from build123d import *

# Parameters (mm, degrees)
SKETCH2_W           = 350.52
SKETCH2_H           = 101.6
SKETCH2_R           = 43.18
SKETCH2_R_2         = 17.78
BOSS_EXTRUDE1_DEPTH = 15.24
SKETCH2_3_R         = 43.18
SKETCH2_3_R_2       = 20.32
BOSS_EXTRUDE2_DEPTH = 10.16
BOSS_EXTRUDE3_START = -50.8
BOSS_EXTRUDE3_DEPTH = 12.7
BOSS_EXTRUDE4_START = 50.8
BOSS_EXTRUDE4_DEPTH = 12.7
FILLET1_R           = 30.48


with BuildPart() as part:
    # Sketch2 → Boss-Extrude1 (new body)
    with BuildSketch(Plane(origin=(0, 0, 0), x_dir=(1, 0, 0), z_dir=(0, 1, 0))):
        Rectangle(SKETCH2_W, SKETCH2_H)
        Circle(SKETCH2_R, mode=Mode.SUBTRACT)
        with Locations((128.27, 0)):
            Circle(SKETCH2_R_2, mode=Mode.SUBTRACT)
        with Locations((-128.27, 0)):
            Circle(SKETCH2_R_2, mode=Mode.SUBTRACT)
    extrude(amount=BOSS_EXTRUDE1_DEPTH)

    # Sketch2<3> → Boss-Extrude2 (add)
    with BuildSketch(Plane(origin=(0, 0, 0), x_dir=(1, 0, 0), z_dir=(0, 1, 0))):
        Circle(SKETCH2_3_R)
        Circle(SKETCH2_3_R_2, mode=Mode.SUBTRACT)
    extrude(amount=BOSS_EXTRUDE2_DEPTH)

    # Sketch3 → Revolve1 (revolve)
    with BuildSketch(Plane.XY):
        Polygon((43.18, 15.24), (43.18, 0), (81.28, 0), (81.28, 101.6), (73.66, 101.6), (73.66, 96.52), (55.88, 96.52), (55.88, 71.12), (68.58, 71.12), (68.58, 15.24), align=None)
    revolve(axis=Axis((0, 0, 0), (0, 1, 0)))

    # Sketch4 → Boss-Extrude3 (add)
    with BuildSketch(Plane.XY.offset(BOSS_EXTRUDE3_START)):
        Polygon((119.38, 15.24), (63.297160251, 101.6), (63.297160251, 15.24), align=None)
        Polygon((-63.297160251, 15.24), (-119.38, 15.24), (-63.297160251, 101.6), align=None)
    extrude(amount=BOSS_EXTRUDE3_DEPTH)

    # Sketch4<2> → Boss-Extrude4 (add)
    with BuildSketch(Plane.XY.offset(BOSS_EXTRUDE4_START)):
        Polygon((119.38, 15.24), (63.297160251, 101.6), (63.297160251, 15.24), align=None)
        Polygon((-63.297160251, 15.24), (-119.38, 15.24), (-63.297160251, 101.6), align=None)
    extrude(amount=-BOSS_EXTRUDE4_DEPTH)

    # Fillet1
    fillet1_edges = [part.edges().sort_by_distance(p)[0] for p in [
        (-175.26, 7.62, 50.8),
        (-175.26, 7.62, -50.8),
        (175.26, 7.62, -50.8),
        (175.26, 7.62, 50.8),
    ]]
    fillet(fillet1_edges, radius=FILLET1_R)


solid = part.part
Model file for the job. Use its own axes, mm. A direction names the side the tool comes from. Give positions to 0.01 mm unless a question says otherwise; leave off trailing zeros. Loops run counter-clockwise (first coordinate to the right, second up) from the corner with the lowest first, then second, coordinate; pieces in that order, holes last.
Item 1: Drop flat-ended pins along their axis: P1, Ø3, axis at x = -58, y = 54, coming from the +Z side; P2, Ø5, axis at y = 73, z = -37.5, coming from the +X side; P3, Ø24.5, axis at x = -106, y = 27, coming from the +Z side. Give the stop position or say it passes through.
Check values:
P1: stops at z = 58.43
P2: stops at x = 83.45
P3: stops at z = 50.8
Item 2: Slice it at B-B (y = 34.5). Write the cut outline in (x, z).
Check values:
outline: (-106.87, -50.8) - (-63.45, -50.8) arc R81.28 ccw to (63.45, -50.8) - (106.87, -50.8) - (106.87, -38.1) - (71.8, -38.1) arc R81.28 ccw to (71.8, 38.1) - (106.87, 38.1) - (106.87, 50.8) - (63.45, 50.8) arc R81.28 ccw to (-63.45, 50.8) - (-106.87, 50.8) - (-106.87, 38.1) - (-71.8, 38.1) arc R81.28 ccw to (-71.8, -38.1) - (-106.87, -38.1) - close; hole circle Ø137.16 at (0, 0)
Item 3: Slice it at D-D (x = 127.5). Write the cut outline in (y, z).
Check values:
outline: (0, -50.8) - (15.24, -50.8) - (15.24, -17.76) - (0, -17.76) - close; (0, 17.76) - (15.24, 17.76) - (15.24, 50.8) - (0, 50.8) - close
Item 4: Slice it at C-C (z = -61). Write the cut outline in (x, y), plus the area to 3 significant figures.
Check values:
outline: (-53.72, 0) - (53.72, 0) - (53.72, 101.6) - (41.29, 101.6) - (41.29, 96.52) - (-41.29, 96.52) - (-41.29, 101.6) - (-53.72, 101.6) - close; hole (-31.34, 15.24) - (31.34, 15.24) - (31.34, 71.12) - (-31.34, 71.12) - close
area: 6,990 mm2
Item 5: Drill centre lines: line 1 along Z through (x, y) = (0, 84); line 2 along Z through (x, y) = (0, 48). Where is each one in solid material? Low to high.
Check values:
line 1: z = -81.28 to -55.88, 55.88 to 81.28
line 2: z = -81.28 to -68.58, 68.58 to 81.28
Item 6: Mould opens along Y. For faces 4 (the face through (-147, 15.24, -1)), 5 (the face through (56.2, 71.12, -0.3)), 6 (the face through (-111.846, 7.513, 6.81)) say: +Y half, -Y half, draft (parallel to the pull), parting line (faces both ways), or undercut.
Check values:
face 4: +Y half
face 5: undercut
face 6: draft
Item 7: Slice it at A-A (x = 0). Write the cut outline in (y, z).
Check values:
outline: (0, -81.28) - (101.6, -81.28) - (101.6, -73.66) - (96.52, -73.66) - (96.52, -55.88) - (71.12, -55.88) - (71.12, -68.58) - (15.24, -68.58) - (15.24, -43.18) - (10.16, -43.18) - (10.16, -20.32) - (0, -20.32) - close; (0, 20.32) - (10.16, 20.32) - (10.16, 43.18) - (15.24, 43.18) - (15.24, 68.58) - (71.12, 68.58) - (71.12, 55.88) - (96.52, 55.88) - (96.52, 73.66) - (101.6, 73.66) - (101.6, 81.28) - (0, 81.28) - close
Item 8: Which spindle directions (+Z, -Z, +X, -X, +Y, -Y) get a long thin tool onto all of the face, cutting with end or side? Do faces 1 (the face through (36.868, 42.789, -57.827)), 2 (the face through (-85, 29, -50.8)), 3 (the face through (-87, 27, 50.8)). Say none if no direction does.
Check values:
face 1: none
face 2: -Z, -X, +Y, -Y
face 3: +Z, -X, +Y, -Y
